Here's how the part is built. I have some questions about the finished solid (model axes, mm). Face numbers are marked on the shaded views. A direction names the side the tool comes from. Round coordinates to 2 decimals unless told otherwise and drop trailing zeros. Write each loop counter-clockwise with the first axis right and the second up, starting at its lowest first coordinate (ties: lowest second). Pieces come first, ordered by that corner, then holes. Notation, with made-up numbers: M 56,21 L 102,21 A28 cw 102,52 Z; hole C 9.25,80.5 d2. An arc over 180 degrees is marked long. Write item = value, one per line. Start each with the question number.
(1) If we mould it in two halves opening along X, with no side actions, what happens to the marked faces 1, 2 and 3? For each: released by +X, released by -X, zero draft, split by the parting line, or undercut.
(2) Will these pins go through, and if not, where does the flat tip stop? pin 1 Ø1.8 at (y, z) = (5.5, 3.5) entering from -X; pin 2 Ø3.5 at (x, z) = (-18.879, 3) entering from -Y; pin 3 Ø1.8 at (y, z) = (3, 1.5) entering from +X.
(3) I want a section at B-B (y = 6.75). List the corners of the cut face in (x, z) for me, and give its area (3 significant figures).
(4) I want a section at A-A (z = 3). List the corners of the cut face in (x, y) for me, and give its area (3 significant figures).
(5) I need wall thicknesses on line 1 along X through (y, z) = (11.35, 3); line 2 along X through (y, z) = (4.5, 1.9); line 3 along Y through (x, z) = (-18, 0.6). Which ranges of each line are inside material? Lowest first, please.
(6) I want a section at C-C (x = -18). List the corners of the cut face in (y, z) for me.
(7) I want a section at D-D (z = 5.2). List the corners of the cut face in (x, y) for me.
(8) On a 3-axis mill with a long thin cutter (end or side, diameter ignored), from which of +Z, -Z, +X, -X, +Y, -Y can I reach the whole of each face in a straight line? I mean the marked faces 4 and 5. Say none if no direction works.
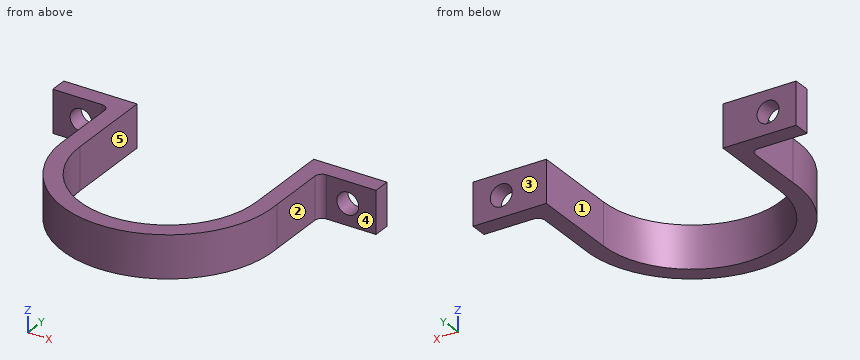
Autodesk Inventor part; units mm, degrees
ref_plane "YZ Plane" through (0, 0, 0) normal (1, 0, 0) x (0, 1, 0)
ref_plane "XZ Plane" through (0, 0, 0) normal (0, 1, 0) x (-1, 0, 0)
ref_plane "XY Plane" through (0, 0, 0) normal (0, 0, 1) x (1, 0, 0)
sketch "Sketch1" plane through (0, 0, 0) normal (0, 0, 1) x (1, 0, 0)
  arc A0 (-12.5, 0) -> (12.5, 0) centre (0, 0) ccw
  line L0 (-12.5, 0) -> (-12.5, 12.5)
  line L1 (12.5, 0) -> (12.5, 12.5)
  arc A1 (-14.879, 0.7912) -> (14.879, 0.7912) centre (0, 0) ccw
  line L2 (-14.879, 0.7912) -> (-14.879, 10.1)
  line L3 (14.879, 0.7912) -> (14.879, 10.1)
  line L4 (-22.879, 12.5) -> (-22.879, 10.1)
  line L5 (-22.879, 10.1) -> (-14.879, 10.1)
  line L6 (-22.879, 12.5) -> (-12.5, 12.5)
  line L7 (22.879, 12.5) -> (22.879, 10.1)
  line L8 (22.879, 10.1) -> (14.879, 10.1)
  line L9 (22.879, 12.5) -> (12.5, 12.5)
extrude "Extrusion1" add sketch "Sketch1" along normal blind 6
sketch "Sketch2" plane through (12.5, 12.5, 0) normal (0, 1, 0) x (1, 0, 0)
  line L0 (-35.379, 0) -> (-35.379, -6)
  circle A0 centre (-31.379, -3) radius 1.55
  circle A1 centre (6.379, -3) radius 1.55
  line L1 (10.379, 0) -> (10.379, -6)
  point P0 (-12.5, 0)
  dimension "d16" = 3.1
extrude "Extrusion2" cut sketch "Sketch2" against normal blind 10
fillet "Fillet1" radius 1 1 edges at (14.879, 10.1, 3)
fillet "Fillet2" radius 1 1 edges at (-14.879, 10.1, 3)
properties part number "motor_support"
Returned:
q1.face_1 = undercut
q1.face_2 = released by +X
q1.face_3 = zero draft
q2.pin_1 = -14.88
q2.pin_2 = 10.1
q2.pin_3 = 14.88
q3.outline = M -14.88,0 L -12.5,0 L -12.5,6 L -14.88,6 Z; M 12.5,0 L 14.88,0 L 14.88,6 L 12.5,6 Z
q3.area = 28.5 mm²
q4.outline = M -22.88,10.1 L -20.43,10.1 L -20.43,12.5 L -22.88,12.5 Z; M -17.33,10.1 L -15.88,10.1 A1 cw -14.88,9.1 L -14.88,0.79 A14.9 ccw long 14.88,0.79 L 14.88,9.1 A1 cw 15.88,10.1 L 17.33,10.1 L 17.33,12.5 L 12.5,12.5 L 12.5,0 A12.5 cw -12.5,0 L -12.5,12.5 L -17.33,12.5 Z; M 20.43,10.1 L 22.88,10.1 L 22.88,12.5 L 20.43,12.5 Z
q4.area = 187 mm²
q5.line_1 = -22.88 to -20.43, -17.33 to -12.5, 12.5 to 17.33, 20.43 to 22.88
q5.line_2 = -14.88 to -12.5, 12.5 to 14.88
q5.line_3 = 10.1 to 12.5
q6.outline = M 10.1,0 L 12.5,0 L 12.5,1.72 L 10.1,1.72 Z; M 10.1,4.28 L 12.5,4.28 L 12.5,6 L 10.1,6 Z
q7.outline = M -22.88,10.1 L -15.88,10.1 A1 cw -14.88,9.1 L -14.88,0.79 A14.9 ccw long 14.88,0.79 L 14.88,9.1 A1 cw 15.88,10.1 L 22.88,10.1 L 22.88,12.5 L 12.5,12.5 L 12.5,0 A12.5 cw -12.5,0 L -12.5,12.5 L -22.88,12.5 Z
q8.face_4 = +Z, -Z, +X, -Y
q8.face_5 = +Z, -Z, +Y
